Could you check a few things on this model? Use its own coordinates, in mm. A direction names the side the tool comes from. Round coordinates to 2 decimals unless told otherwise and drop trailing zeros. Loops run counter-clockwise (first coordinate to the right, second up) from the corner with the lowest first, then second, coordinate; pieces in that order, holes last. Notation, with made-up numbers: (54, -1) -> (93, -1) arc R17 ccw to (93, 23) -> close; hole circle Ø11 at (-10.75, -9.75). An arc over 180 degrees is marked (long way). One line per item, written item: value.
```python
from build123d import *

# Parameters (mm, degrees)
F0_W     = 4.4881204973
F0_H     = 1
F0_W_2   = 1
F0_H_2   = 9.6190602487
F0_H_3   = 7.107180746
F1_DEPTH = 8.65
F2_DEPTH = 5
F3_DEPTH = 5
F5_DEPTH = 3.65
F6_R     = 1.5
F7_DEPTH = 3.65


with BuildPart() as f1:
    # F0 (on Front) → F1 (new body)
    with BuildSketch(Plane.XZ):
        with BuildLine():
            Line((34.3548780517, 39.6712920324), (6.5856519265, 67.4405181576))
            Line((6.5856519265, 67.4405181576), (-66.2696871329, -5.4148209018))
            Line((-66.2696871329, -5.4148209018), (-38.5004610077, -33.1840470269))
            add(Edge.make_bspline(
                [(-38.5004610077, -33.1840470269), (-38.1234667087, -33.490568944), (-37.3694781107, -34.1036127783), (-36.4028402078, -34.2032757765), (-35.9195212563, -34.2531072756)],
                knots=[0, 0, 0, 0, 0.5, 1, 1, 1, 1], degree=3))
            Line((-35.9195212563, -34.2531072756), (-1.4432802617, -34.2531072756))
            add(Edge.make_bspline(
                [(-1.4432802617, -34.2531072756), (-0.9599613102, -34.2032757765), (0.0066765927, -34.1036127783), (0.7606651907, -33.490568944), (1.1376594897, -33.1840470269)],
                knots=[0, 0, 0, 0, 0.5, 1, 1, 1, 1], degree=3))
            Line((1.1376594897, -33.1840470269), (17.7462687707, -16.5754377459))
            Line((17.7462687707, -16.5754377459), (34.3548780517, 0.0331715351))
            add(Edge.make_bspline(
                [(34.3548780517, 0.0331715351), (34.6613999688, 0.4101658341), (35.274443803, 1.164154432), (35.3741068012, 2.1307923349), (35.4239383003, 2.6141112864)],
                knots=[0, 0, 0, 0, 0.5, 1, 1, 1, 1], degree=3))
            Line((35.4239383003, 2.6141112864), (35.4239383003, 37.0903522811))
            add(Edge.make_bspline(
                [(35.4239383003, 37.0903522811), (35.3741068012, 37.5736712325), (35.274443803, 38.5403091354), (34.6613999688, 39.2942977334), (34.3548780517, 39.6712920324)],
                knots=[0, 0, 0, 0, 0.5, 1, 1, 1, 1], degree=3))
        make_face()
        Polygon((-61.8149144114, -6.1219276829), (-37.3337348187, -30.6031072756), (-38.0408415999, -31.3102140568), (-62.5220211925, -6.8290344641), align=None, mode=Mode.SUBTRACT)
        with Locations((-32.6754610077, -32.1031072756)):
            Rectangle(F0_W, F0_H, mode=Mode.SUBTRACT)
        with Locations((-4.6873405103, -32.1031072756)):
            Rectangle(F0_W, F0_H, mode=Mode.SUBTRACT)
        Polygon((5.6193874733, -24.954653103), (6.3264942545, -25.6617598842), (0.6780400819, -31.3102140568), (-0.0290666993, -30.6031072756), align=None, mode=Mode.SUBTRACT)
        Polygon((25.4183773465, -3.7414496674), (15.1653290193, -13.9944979946), (-0.7361734805, -29.8960004944), (-2.4432802617, -30.6031072756), (-6.931400759, -30.6031072756), (-30.431400759, -30.6031072756), (-34.9195212563, -30.6031072756), (-36.6266280375, -29.8960004944), (-61.1078076302, -5.4148209018), (6.5856519265, 62.2786386549), (31.0668315191, 37.7974590623), (31.7739383003, 36.0903522811), (31.7739383003, 3.6141112864), (31.0668315191, 1.9070045052), align=None, mode=Mode.SUBTRACT)
        Polygon((32.4810450815, 0.4927909428), (26.8325909089, -5.1556632298), (26.1254841277, -4.4485564486), (31.7739383003, 1.199897724), align=None, mode=Mode.SUBTRACT)
        with Locations((33.2739383003, 8.4236414107)):
            Rectangle(F0_W_2, F0_H_2, mode=Mode.SUBTRACT)
        Polygon((-62.5220211926, -4.0006073394), (5.1714383642, 63.6928522173), (5.8785451453, 62.9857454361), (-61.8149144114, -4.7077141206), align=None, mode=Mode.SUBTRACT)
        with Locations((33.2739383003, 32.5367619081)):
            Rectangle(F0_W_2, F0_H_3, mode=Mode.SUBTRACT)
        Polygon((7.9998654889, 63.6928522172), (32.4810450815, 39.2116726246), (31.7739383003, 38.5045658435), (7.2927587077, 62.9857454361), align=None, mode=Mode.SUBTRACT)
        Polygon((-0.7361734805, -29.8960004944), (15.1653290193, -13.9944979946), (25.4183773465, -3.7414496674), (31.0668315191, 1.9070045052), (31.7739383003, 3.6141112864), (31.7739383003, 36.0903522811), (31.0668315191, 37.7974590623), (6.5856519265, 62.2786386549), (-61.1078076302, -5.4148209018), (-36.6266280375, -29.8960004944), (-34.9195212563, -30.6031072756), (-30.431400759, -30.6031072756), (-6.931400759, -30.6031072756), (-2.4432802617, -30.6031072756), align=None)
        Polygon((5.8785451453, 62.9857454361), (5.1714383642, 63.6928522173), (-62.5220211926, -4.0006073394), (-61.8149144114, -4.7077141206), align=None)
        Polygon((31.7739383003, 38.5045658435), (32.4810450815, 39.2116726246), (7.9998654889, 63.6928522172), (7.2927587077, 62.9857454361), align=None)
        Polygon((-38.0408415999, -31.3102140568), (-37.3337348187, -30.6031072756), (-61.8149144114, -6.1219276829), (-62.5220211925, -6.8290344641), align=None)
        with Locations((33.2739383003, 8.4236414107)):
            Rectangle(F0_W_2, F0_H_2)
        Polygon((26.1254841277, -4.4485564486), (26.8325909089, -5.1556632298), (32.4810450815, 0.4927909428), (31.7739383003, 1.199897724), align=None)
        Polygon((0.6780400819, -31.3102140568), (6.3264942545, -25.6617598842), (5.6193874733, -24.954653103), (-0.0290666993, -30.6031072756), align=None)
        with Locations((33.2739383003, 32.5367619081)):
            Rectangle(F0_W_2, F0_H_3)
        with Locations((-4.6873405103, -32.1031072756)):
            Rectangle(F0_W, F0_H)
        with Locations((-32.6754610077, -32.1031072756)):
            Rectangle(F0_W, F0_H)
    extrude(amount=F1_DEPTH)

    # F0 (on Front) → F2 (cut)
    with BuildSketch(Plane.XZ):
        Polygon((-0.7361734805, -29.8960004944), (15.1653290193, -13.9944979946), (25.4183773465, -3.7414496674), (31.0668315191, 1.9070045052), (31.7739383003, 3.6141112864), (31.7739383003, 36.0903522811), (31.0668315191, 37.7974590623), (6.5856519265, 62.2786386549), (-61.1078076302, -5.4148209018), (-36.6266280375, -29.8960004944), (-34.9195212563, -30.6031072756), (-30.431400759, -30.6031072756), (-6.931400759, -30.6031072756), (-2.4432802617, -30.6031072756), align=None)
    extrude(amount=F2_DEPTH, mode=Mode.SUBTRACT)

    # F0 (on Front) → F3 (cut)
    with BuildSketch(Plane.XZ):
        Polygon((31.7739383003, 38.5045658435), (32.4810450815, 39.2116726246), (7.9998654889, 63.6928522172), (7.2927587077, 62.9857454361), align=None)
        Polygon((5.8785451453, 62.9857454361), (5.1714383642, 63.6928522173), (-62.5220211926, -4.0006073394), (-61.8149144114, -4.7077141206), align=None)
        Polygon((-38.0408415999, -31.3102140568), (-37.3337348187, -30.6031072756), (-61.8149144114, -6.1219276829), (-62.5220211925, -6.8290344641), align=None)
        with Locations((-32.6754610077, -32.1031072756)):
            Rectangle(F0_W, F0_H)
        with Locations((-4.6873405103, -32.1031072756)):
            Rectangle(F0_W, F0_H)
        Polygon((0.6780400819, -31.3102140568), (6.3264942545, -25.6617598842), (5.6193874733, -24.954653103), (-0.0290666993, -30.6031072756), align=None)
        Polygon((26.1254841277, -4.4485564486), (26.8325909089, -5.1556632298), (32.4810450815, 0.4927909428), (31.7739383003, 1.199897724), align=None)
        with Locations((33.2739383003, 8.4236414107)):
            Rectangle(F0_W_2, F0_H_2)
        with Locations((33.2739383003, 32.5367619081)):
            Rectangle(F0_W_2, F0_H_3)
    extrude(amount=F3_DEPTH, mode=Mode.SUBTRACT)

    # F4 (on face) → F5 (cut, through all)
    with BuildSketch(Plane(origin=(0, -5, 0), x_dir=(-1, 0, 0), z_dir=(0, 1, 0))):
        Polygon((-3.6387139853, 9.1271192495), (-20.9628301244, -8.1969968896), (-9.2955682348, -19.8642587791), (8.0285479043, -2.5401426401), align=None)
    extrude(amount=-F5_DEPTH, mode=Mode.SUBTRACT)

    # F6 (on face) → F7 (cut, through all)
    with BuildSketch(Plane.XZ.offset(8.65)):
        with Locations((3.4263458096, 39.1169224389)):
            Circle(F6_R)
        with Locations((-36.5514419514, -0.8608653222)):
            Circle(F6_R)
    extrude(amount=-F7_DEPTH, mode=Mode.SUBTRACT)


solid = f1.part
```
Item 1: I need wall thicknesses on line 1 (X direction, y = -1.5, z = -17.5); line 2 (X direction, y = -0.5, z = 9.5); line 3 (Z direction, x = -40.5, y = -2.75). Which ranges of each line are inside material? Lowest first, please. Write a range as from..to.
Output:
line 1: x = -54.18..-51.85, -50.44..-49.02, 11.66..16.82
line 2: x = -51.35..-49.02, -47.61..-46.19, 31.77..32.77, 33.77..35.42
line 3: z = -31.18..-28.85, -27.44..-26.02, 15.19..16.61, 18.02..20.35
Item 2: For faces 1 (the face through (33.774, -2, 32)), 2 (the face through (35.424, -4, 20)), 3 (the face through (0.75, -6.8, -11.32)), which set-ups out of +Z, -Z, +X, -X, +Y, -Y let a thin tool reach every point of the face, with its end or its side?
Output:
face 1: +Y
face 2: +Z, -Z, +X, +Y, -Y
face 3: +Y, -Y
Item 3: Will these pins go through, and if not, where does the flat tip stop? pin 1 Ø0.5 at (x, z) = (-5, -32) entering from +Y; pin 2 Ø0.5 at (x, y) = (33.5, -2) entering from +Z; pin 3 Ø0.8 at (x, y) = (33.5, -3.5) entering from -Z.
Output:
pin 1: stops at y = -5
pin 2: stops at z = 40.78
pin 3: stops at z = -1.22
Item 4: If we section it at D-D on x = -4: List the corners of the cut face in (y, z) for me, plus the area to 3 significant figures.
Output:
outline: (-8.65, -34.25) -> (0, -34.25) -> (0, -32.6) -> (-5, -32.6) -> (-5, -31.6) -> (0, -31.6) -> (0, -30.6) -> (-5, -30.6) -> (-5, -6.57) -> (-8.65, -6.57) -> close; (-8.65, 1.49) -> (-5, 1.49) -> (-5, 51.69) -> (0, 51.69) -> (0, 53.11) -> (-5, 53.11) -> (-5, 54.52) -> (0, 54.52) -> (0, 56.85) -> (-8.65, 56.85) -> close
area: 335 mm²
Item 5: If we section it at C-C on z = 17.5: List the corners of the cut face in (x, y) for me.
Output:
outline: (-43.35, -8.65) -> (35.42, -8.65) -> (35.42, 0) -> (31.77, 0) -> (31.77, -5) -> (-38.19, -5) -> (-38.19, 0) -> (-39.61, 0) -> (-39.61, -5) -> (-41.02, -5) -> (-41.02, 0) -> (-43.35, 0) -> close
Item 6: If we section it at A-A on z = -14: List the corners of the cut face in (x, y) for me, plus the area to 3 significant figures.
Output:
outline: (-57.68, -8.65) -> (3.43, -8.65) -> (3.43, -5) -> (-52.52, -5) -> (-52.52, 0) -> (-53.94, 0) -> (-53.94, -5) -> (-55.35, -5) -> (-55.35, 0) -> (-57.68, 0) -> close; (15.16, -8.65) -> (20.32, -8.65) -> (20.32, 0) -> (15.16, 0) -> close
area: 286 mm²
Item 7: If we section it at B-B on x = -48: List the corners of the cut face in (y, z) for me.
Output:
outline: (-8.65, -23.68) -> (0, -23.68) -> (0, -21.35) -> (-5, -21.35) -> (-5, -19.94) -> (0, -19.94) -> (0, -18.52) -> (-5, -18.52) -> (-5, 7.69) -> (0, 7.69) -> (0, 9.11) -> (-5, 9.11) -> (-5, 10.52) -> (0, 10.52) -> (0, 12.85) -> (-8.65, 12.85) -> close
